Read the model definition and answer for the solid it produces. Units are mm, in the model's axes. Face numbers are marked on the shaded views. A direction names the side the tool comes from. Give positions to 0.01 mm unless a question says otherwise; leave off trailing zeros. Order: outer loops, then holes, each group sorted by start corner. A loop starts at its lowest first (then second) coordinate and runs counter-clockwise, first axis right, second up. Notation, with made-up numbers: (33.25, 22) - (57.25, 22) arc R38 ccw to (57.25, 60) - close; hole circle Ø2 at (2, 32). An arc over 180 degrees is marked (long way). Write each question's results on one line, items separated by ' | '.
from build123d import *

# Parameters (mm, degrees)
ESBO_O1_R                = 10
RESSALTO_EXTRUS_O1_DEPTH = 12.5
CAVIDADE1_START          = -12.5
CAVIDADE1_DEPTH          = 25


# Read off the part's stored shape, not the designer's step: Cavidade1
with BuildPart() as part:
    # Esboço1 → Ressalto-extrusão1 (new, symmetric)
    with BuildSketch(Plane.XY):
        Circle(ESBO_O1_R)
    extrude(amount=RESSALTO_EXTRUS_O1_DEPTH, both=True)

    # Cavidade1 outline → Cavidade1 (cut)
    with BuildSketch(Plane.XY.offset(CAVIDADE1_START)):
        with BuildLine():
            Line((4.446152423, 4.299038106), (4.821152423, 3.649519053))
            Line((4.821152423, 3.649519053), (6.087632977, 4.380721942))
            ThreePointArc((6.087632977, 4.380721942), (3.75, 6.495190528), (0.75, 7.462405778))
            Line((0.75, 7.462405778), (0.75, 6))
            Line((0.75, 6), (1.5, 6))
            Line((1.5, 6), (1.5, 4.5))
            Line((1.5, 4.5), (-1.5, 4.5))
            Line((-1.5, 4.5), (-1.5, 6))
            Line((-1.5, 6), (-0.75, 6))
            Line((-0.75, 6), (-0.75, 7.462405778))
            ThreePointArc((-0.75, 7.462405778), (-3.75, 6.495190528), (-6.087632977, 4.380721942))
            Line((-6.087632977, 4.380721942), (-4.821152423, 3.649519053))
            Line((-4.821152423, 3.649519053), (-4.446152423, 4.299038106))
            Line((-4.446152423, 4.299038106), (-3.147114317, 3.549038106))
            Line((-3.147114317, 3.549038106), (-4.647114317, 0.950961894))
            Line((-4.647114317, 0.950961894), (-5.946152423, 1.700961894))
            Line((-5.946152423, 1.700961894), (-5.571152423, 2.350480947))
            Line((-5.571152423, 2.350480947), (-6.837632977, 3.081683836))
            ThreePointArc((-6.837632977, 3.081683836), (-7.5, 0), (-6.837632977, -3.081683836))
            Line((-6.837632977, -3.081683836), (-5.571152423, -2.350480947))
            Line((-5.571152423, -2.350480947), (-5.946152423, -1.700961894))
            Line((-5.946152423, -1.700961894), (-4.647114317, -0.950961894))
            Line((-4.647114317, -0.950961894), (-3.147114317, -3.549038106))
            Line((-3.147114317, -3.549038106), (-4.446152423, -4.299038106))
            Line((-4.446152423, -4.299038106), (-4.821152423, -3.649519053))
            Line((-4.821152423, -3.649519053), (-6.087632977, -4.380721942))
            ThreePointArc((-6.087632977, -4.380721942), (-3.75, -6.495190528), (-0.75, -7.462405778))
            Line((-0.75, -7.462405778), (-0.75, -6))
            Line((-0.75, -6), (-1.5, -6))
            Line((-1.5, -6), (-1.5, -4.5))
            Line((-1.5, -4.5), (1.5, -4.5))
            Line((1.5, -4.5), (1.5, -6))
            Line((1.5, -6), (0.75, -6))
            Line((0.75, -6), (0.75, -7.462405778))
            ThreePointArc((0.75, -7.462405778), (3.75, -6.495190528), (6.087632977, -4.380721942))
            Line((6.087632977, -4.380721942), (4.821152423, -3.649519053))
            Line((4.821152423, -3.649519053), (4.446152423, -4.299038106))
            Line((4.446152423, -4.299038106), (3.147114317, -3.549038106))
            Line((3.147114317, -3.549038106), (4.647114317, -0.950961894))
            Line((4.647114317, -0.950961894), (5.946152423, -1.700961894))
            Line((5.946152423, -1.700961894), (5.571152423, -2.350480947))
            Line((5.571152423, -2.350480947), (6.837632977, -3.081683836))
            ThreePointArc((6.837632977, -3.081683836), (7.5, 0), (6.837632977, 3.081683836))
            Line((6.837632977, 3.081683836), (5.571152423, 2.350480947))
            Line((5.571152423, 2.350480947), (5.946152423, 1.700961894))
            Line((5.946152423, 1.700961894), (4.647114317, 0.950961894))
            Line((4.647114317, 0.950961894), (3.147114317, 3.549038106))
            Line((3.147114317, 3.549038106), (4.446152423, 4.299038106))
        make_face()
    extrude(amount=CAVIDADE1_DEPTH, mode=Mode.SUBTRACT)


solid = part.part
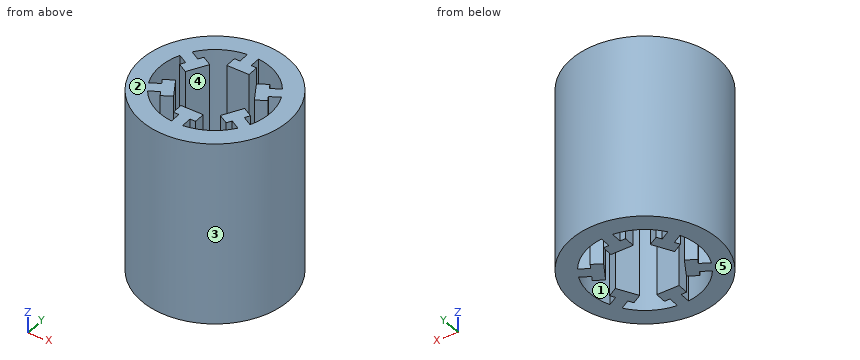
(1) Section A-A (y = 0) is taken. Give the vertices of the cut face in (x, z).
Conclusion:
outline: (-10, -12.5) - (-7.5, -12.5) - (-7.5, 12.5) - (-10, 12.5) - close; (7.5, -12.5) - (10, -12.5) - (10, 12.5) - (7.5, 12.5) - close
(2) The mould has two halves that part along X. Classify the marked faces 1, 2 and 3: pulls with the +X half, pulls with the -X half, needs draft (parallel to the pull), parting line crosses it, or undercut.
Conclusion:
face 1: undercut | face 2: needs draft | face 3: parting line crosses it
(3) Section D-D (y = -2.75) is taken. Give the vertices of the cut face in (x, z).
Conclusion:
outline: (-9.61, -12.5) - (-6.98, -12.5) - (-6.98, 12.5) - (-9.61, 12.5) - close; (-6.26, -12.5) - (-3.61, -12.5) - (-3.61, 12.5) - (-6.26, 12.5) - close; (3.61, -12.5) - (6.26, -12.5) - (6.26, 12.5) - (3.61, 12.5) - close; (6.98, -12.5) - (9.61, -12.5) - (9.61, 12.5) - (6.98, 12.5) - close
(4) Each of these flat-tipped pins is pushed along its axis until it touches: pin 1 (1.5 mm diameter, centred on y = -2, z = 5.5, fed in from +X); pin 2 (1 mm diameter, centred on x = 1.5, z = -4, fed in from -Y); pin 3 (1.5 mm diameter, centred on x = -6.5, z = -1, fed in from -Y). Where does it stop, or does it pass through?
Conclusion:
pin 1: x = 9.92 | pin 2: y = -9.95 | pin 3: y = -8.18
(5) For the marked faces 4 and 5, determine the directions among +Z, -Z, +X, -X, +Y, -Y from which every point of the face is accessible in a straight line to the end or side of a thin tool.
Conclusion:
face 4: +Z, -Z | face 5: -Z, +X, -X, +Y, -Y
(6) Section C-C (x = -3.5) is taken. Give the vertices of the cut face in (y, z), plus the area to 3 significant figures.
Conclusion:
outline: (-9.37, -12.5) - (-6.63, -12.5) - (-6.63, 12.5) - (-9.37, 12.5) - close; (-3.75, -12.5) - (-2.94, -12.5) - (-2.94, 12.5) - (-3.75, 12.5) - close; (2.94, -12.5) - (3.75, -12.5) - (3.75, 12.5) - (2.94, 12.5) - close; (6.63, -12.5) - (9.37, -12.5) - (9.37, 12.5) - (6.63, 12.5) - close | area: 177 mm^2
(7) Consider probe 1 along X at (y, z) = (-6.75, -7.75); probe 2 along X at (y, z) = (0.25, -5.25); probe 3 along X at (y, z) = (2.25, 5.25). Determine where each line is inside the solid, lowest interval first. Write a range as [from, to].
Conclusion:
probe 1: [-7.38, -3.27], [-0.75, 0.75], [3.27, 7.38] | probe 2: [-10, -7.5], [7.5, 10] | probe 3: [-9.74, -7.15], [-5.63, -3.9], [3.9, 5.63], [7.15, 9.74]
(8) Section B-B (x = 0) is taken. Give the vertices of the cut face in (y, z), plus the area to 3 significant figures.
Conclusion:
outline: (-10, -12.5) - (-4.5, -12.5) - (-4.5, 12.5) - (-10, 12.5) - close; (4.5, -12.5) - (10, -12.5) - (10, 12.5) - (4.5, 12.5) - close | area: 275 mm^2
